```python
from build123d import *

# Parameters (mm, degrees)
SKETCH2_R           = 1.7
BOSS_EXTRUDE1_DEPTH = 1
BOSS_EXTRUDE2_START = -3
BOSS_EXTRUDE2_DEPTH = 3


with BuildPart() as part:
    # Sketch2 → Boss-Extrude1 (new body)
    with BuildSketch(Plane.XY):
        with BuildLine():
            Line((28.78011557, -21.498473491), (21.333027704, -14.051385626))
            ThreePointArc((21.333027704, -14.051385626), (20.684181007, -13.617840123), (19.918814142, -13.465599188))
            Line((19.918814142, -13.465599188), (-4.3, -13.465599188))
            ThreePointArc((-4.3, -13.465599188), (-6.421320344, -14.344278845), (-7.3, -16.465599188))
            Line((-7.3, -16.465599188), (-7.3, -99.073599188))
            ThreePointArc((-7.3, -99.073599188), (-6.421320344, -101.194919532), (-4.3, -102.073599188))
            Line((-4.3, -102.073599188), (19.918814142, -102.073599188))
            ThreePointArc((19.918814142, -102.073599188), (20.684181007, -101.921358253), (21.333027704, -101.48781275))
            Line((21.333027704, -101.48781275), (28.78511557, -94.035724885))
            ThreePointArc((28.78511557, -94.035724885), (32.741782732, -91.39196441), (37.408989873, -90.463599188))
            Line((37.408989873, -90.463599188), (107.834, -90.463599188))
            ThreePointArc((107.834, -90.463599188), (108.841627163, -90.046226351), (109.259, -89.038599188))
            Line((109.259, -89.038599188), (109.259, -26.495599188))
            ThreePointArc((109.259, -26.495599188), (108.841627163, -25.487972025), (107.834, -25.070599188))
            Line((107.834, -25.070599188), (37.403989873, -25.070599188))
            ThreePointArc((37.403989873, -25.070599188), (32.736782732, -24.142233967), (28.78011557, -21.498473491))
        make_face()
        with Locations((106.406, -27.923599188)):
            Circle(SKETCH2_R, mode=Mode.SUBTRACT)
        with Locations((19.565489973, -16.318599188)):
            Circle(SKETCH2_R, mode=Mode.SUBTRACT)
        with Locations((-4.447, -16.318599188)):
            Circle(SKETCH2_R, mode=Mode.SUBTRACT)
        with Locations((-4.447, -99.220599188)):
            Circle(SKETCH2_R, mode=Mode.SUBTRACT)
        with Locations((19.565489973, -99.220599188)):
            Circle(SKETCH2_R, mode=Mode.SUBTRACT)
        with Locations((106.406, -87.610599188)):
            Circle(SKETCH2_R, mode=Mode.SUBTRACT)
        with BuildLine():
            Line((15.815448907, -99.369599188), (3, -99.369599188))
            ThreePointArc((3, -99.369599188), (1.51507576, -98.754523429), (0.9, -97.269599188))
            Line((0.9, -97.269599188), (0.9, -18.269599188))
            ThreePointArc((0.9, -18.269599188), (1.51507576, -16.784674948), (3, -16.169599188))
            Line((3, -16.169599188), (15.815448907, -16.169599188))
            ThreePointArc((15.815448907, -16.169599188), (18.129279051, -19.785919074), (22.322528351, -18.864919746))
            Line((22.322528351, -18.864919746), (31.232207794, -27.774599188))
            Line((31.232207794, -27.774599188), (102.655958934, -27.774599188))
            ThreePointArc((102.655958934, -27.774599188), (103.75222825, -30.577370938), (106.555, -31.673640255))
            Line((106.555, -31.673640255), (106.555, -83.860558122))
            ThreePointArc((106.555, -83.860558122), (103.75222825, -84.956827438), (102.655958934, -87.759599188))
            Line((102.655958934, -87.759599188), (31.237207794, -87.759599188))
            Line((31.237207794, -87.759599188), (22.322528351, -96.674278631))
            ThreePointArc((22.322528351, -96.674278631), (18.129279051, -95.753279303), (15.815448907, -99.369599188))
        make_face(mode=Mode.SUBTRACT)
    extrude(amount=BOSS_EXTRUDE1_DEPTH)

    # Sketch3 → Boss-Extrude2 (add)
    with BuildSketch(Plane.XY.offset(BOSS_EXTRUDE2_START)):
        with BuildLine():
            Line((31.605, -26.874599188), (103.75284942, -26.874599188))
            ThreePointArc((103.75284942, -26.874599188), (104.388624353, -29.940974835), (107.455, -30.576749768))
            Line((107.455, -30.576749768), (107.455, -84.957448608))
            ThreePointArc((107.455, -84.957448608), (104.388624353, -85.593223541), (103.75284942, -88.659599188))
            Line((103.75284942, -88.659599188), (31.61, -88.659599188))
            Line((31.61, -88.659599188), (22.183305753, -98.086293435))
            ThreePointArc((22.183305753, -98.086293435), (18.473694141, -96.584770882), (16.912339393, -100.269599188))
            Line((16.912339393, -100.269599188), (3, -100.269599188))
            ThreePointArc((3, -100.269599188), (0.878679656, -99.390919532), (0, -97.269599188))
            Line((0, -97.269599188), (0, -18.269599188))
            ThreePointArc((0, -18.269599188), (0.878679656, -16.148278845), (3, -15.269599188))
            Line((3, -15.269599188), (16.912339393, -15.269599188))
            ThreePointArc((16.912339393, -15.269599188), (18.473694141, -18.954427494), (22.183305753, -17.452904941))
            Line((22.183305753, -17.452904941), (31.605, -26.874599188))
        make_face()
        with BuildLine():
            Line((102.655958934, -27.774599188), (31.232207794, -27.774599188))
            Line((31.232207794, -27.774599188), (22.322528351, -18.864919746))
            ThreePointArc((22.322528351, -18.864919746), (18.129279051, -19.785919074), (15.815448907, -16.169599188))
            Line((15.815448907, -16.169599188), (3, -16.169599188))
            ThreePointArc((3, -16.169599188), (1.51507576, -16.784674948), (0.9, -18.269599188))
            Line((0.9, -18.269599188), (0.9, -97.269599188))
            ThreePointArc((0.9, -97.269599188), (1.51507576, -98.754523429), (3, -99.369599188))
            Line((3, -99.369599188), (15.815448907, -99.369599188))
            ThreePointArc((15.815448907, -99.369599188), (18.129279051, -95.753279303), (22.322528351, -96.674278631))
            Line((22.322528351, -96.674278631), (31.237207794, -87.759599188))
            Line((31.237207794, -87.759599188), (102.655958934, -87.759599188))
            ThreePointArc((102.655958934, -87.759599188), (103.75222825, -84.956827438), (106.555, -83.860558122))
            Line((106.555, -83.860558122), (106.555, -31.673640255))
            ThreePointArc((106.555, -31.673640255), (103.75222825, -30.577370938), (102.655958934, -27.774599188))
        make_face(mode=Mode.SUBTRACT)
    extrude(amount=BOSS_EXTRUDE2_DEPTH)


solid = part.part
```
Verification items for the finished model (mm, model axes). A direction names the side the tool comes from. Round coordinates to 2 decimals unless told otherwise and drop trailing zeros. Order: outer loops, then holes, each group sorted by start corner. A loop starts at its lowest first (then second) coordinate and runs counter-clockwise, first axis right, second up. Notation, with made-up numbers: (-7, 26) - (13, 26) arc R26 cw to (13, 44) - close; hole circle Ø6 at (46.25, 73). An arc over 180 degrees is marked (long way). Use CSV: the item, a comma, the result in double quotes. Start each with the question number.
1) Thickness scan on L1, parallel to Y at x = 101.5, z = -0.95; L2, parallel to Y at x = 10, z = -1.25; L3, parallel to X at y = -68, z = -1 (3 decimals). Record the ranges inside material, lowest first.
2) Go/stop test with flat-tipped pins: P1, Ø2, axis at x = 79.5, z = -0.5, coming from the -Y side; P2, Ø1.2, axis at x = 12, z = -1.5, coming from the +Y side; P3, Ø4, axis at x = 106.41, y = -27.92, coming from the -Z side. Record where each tip stops, or that it passes through.
3) Section check B-B, the plane x = 85. Record the cut outline in (y, z).
4) Access from +Z, -Z, +X, -X, +Y, -Y to the whole of each face (thin tool, end or side, straight path). Record for faces 5 (the cylindrical face through (0.855, -16.172, -1.521)), 6 (the flat face through (68, -88.66, -2)), 7 (the cylindrical face through (0.9, -99.41, -1.52)), 8 (the flat face through (26.84, -23.38, -1.03)).
5) Section check A-A, the plane y = -81.5. Record the cut outline in (x, z) (3 decimals), plus the area to 3 significant figures.
6) Mould release check, pull along X, two halves, no side actions. Record for faces 1 (the cylindrical face through (18.531, -96.562, -1.521)), 2 (the cylindrical face through (103.72, -84.99, -1.03)), 3 (the flat face through (33, -90, 1)), 4 (the flat face through (25.11, -17.83, 0.49)): +X half, -X half, draft (parallel to the pull), parting line (faces both ways), or undercut.
7) Section check C-C, the plane z = -1.3. Record the cut outline in (x, y) (3 decimals), plus the area to 3 significant figures.
Answers:
1,L1,"y = -88.66 to -87.76, -27.77 to -26.87"
1,L2,"y = -100.27 to -99.37, -16.17 to -15.27"
1,L3,"x = 0 to 0.9, 106.555 to 107.455"
2,P1,"stops at y = -90.46"
2,P2,"stops at y = -15.27"
2,P3,"stops at z = 0"
3,outline,"(-90.46, 0) - (-88.66, 0) - (-88.66, -3) - (-87.76, -3) - (-87.76, 1) - (-90.46, 1) - close; (-27.77, -3) - (-26.87, -3) - (-26.87, 0) - (-25.07, 0) - (-25.07, 1) - (-27.77, 1) - close"
4,face 5,"-Z, -X, +Y"
4,face 6,"-Z, +X, -Y"
4,face 7,"-Z, -X, -Y"
4,face 8,"+Z, -Z"
5,outline,"(-7.3, 0) - (0, 0) - (0, -3) - (0.9, -3) - (0.9, 1) - (-7.3, 1) - close; (106.555, -3) - (107.455, -3) - (107.455, 0) - (109.259, 0) - (109.259, 1) - (106.555, 1) - close"
5,area,"16.3 mm²"
6,face 1,"undercut"
6,face 2,"undercut"
6,face 3,"draft"
6,face 4,"+X half"
7,outline,"(0, -97.27) arc R3 ccw to (3, -100.27) - (16.912, -100.27) arc R2.853 cw to (22.183, -98.086) - (31.61, -88.66) - (103.753, -88.66) arc R2.853 cw to (107.455, -84.957) - (107.455, -30.577) arc R2.853 cw to (103.753, -26.875) - (31.605, -26.875) - (22.183, -17.453) arc R2.853 cw to (16.912, -15.27) - (3, -15.27) arc R3 ccw to (0, -18.27) - close; hole (0.9, -97.27) arc R2.1 ccw to (3, -99.37) - (15.815, -99.37) arc R3.753 cw to (22.323, -96.674) - (31.237, -87.76) - (102.656, -87.76) arc R3.753 cw to (106.555, -83.861) - (106.555, -31.674) arc R3.753 cw to (102.656, -27.775) - (31.232, -27.775) - (22.323, -18.865) arc R3.753 cw to (15.815, -16.17) - (3, -16.17) arc R2.1 ccw to (0.9, -18.27) - close"
7,area,"330 mm²"
